Part model, mm, in its own coordinate system. Face numbers are marked on the shaded views. A direction names the side the tool comes from. Give positions to 0.01 mm unless a question says otherwise; leave off trailing zeros. Order: outer loops, then holes, each group sorted by start corner. A loop starts at its lowest first (then second) coordinate and runs counter-clockwise, first axis right, second up. Notation, with made-up numbers: M -30.5,88.25 L -20.5,88.25 A28 cw -20.5,125.25 Z; hole C 55.25,34 d2. An arc over 180 degrees is marked long. One line per question, with ' | ' between items.
```python
from build123d import *

# Parameters (mm, degrees)
SKETCH_1_R             = 5.5
EXTRUDE_1_DEPTH        = 68
CHAMFER_1_SIZE         = 0.5
SKETCH_2_R             = 3.3
EXTRUDE_2_DEPTH        = 8
HOLE_WIZARD_M5_1_D     = 4.2
HOLE_WIZARD_M5_1_DEPTH = 12.4
HOLE_WIZARD_M5_1_TIP   = 1.2618073
CHAMFER_3_SIZE         = 0.5
SKETCH_6_W             = 10
SKETCH_6_H             = 3
CUT_EXTRUDE_1_DEPTH    = 13


# Read off the part's stored shape, not the designer's step: M6 机械螺纹 螺柱1
with BuildPart() as part:
    # 草图1 → 拉伸1 (new body)
    with BuildSketch(Plane.XY):
        Circle(SKETCH_1_R)
    extrude(amount=EXTRUDE_1_DEPTH)

    # 倒角1
    chamfer_1_edges = [part.edges().sort_by_distance(p)[0] for p in [
        (-5.5, 0, 0),
        (-5.5, 0, 68),
    ]]
    chamfer(chamfer_1_edges, length=CHAMFER_1_SIZE)

    # 草图2 → 拉伸2 (add)
    with BuildSketch(Plane.XY.offset(68)):
        Circle(SKETCH_2_R)
    extrude(amount=EXTRUDE_2_DEPTH)

    # M5 螺纹孔1
    with Locations(Plane(origin=(0, 0, 0), x_dir=(-1, 0, 0), z_dir=(0, 0, -1))):
        with Locations((0, 0)):
            Hole(HOLE_WIZARD_M5_1_D / 2, depth=HOLE_WIZARD_M5_1_DEPTH)
            with Locations((0, 0, -(HOLE_WIZARD_M5_1_DEPTH + HOLE_WIZARD_M5_1_TIP / 2))):  # 118° drill point
                Cone(0, HOLE_WIZARD_M5_1_D / 2, HOLE_WIZARD_M5_1_TIP, mode=Mode.SUBTRACT)

    # 倒角3
    chamfer_3_edges = [part.edges().sort_by_distance(p)[0] for p in [
        (-2.1, 0, 0),
    ]]
    chamfer(chamfer_3_edges, length=CHAMFER_3_SIZE)

    # 草图6 → 切除-拉伸1 (cut)
    with BuildSketch(Plane(origin=(0, 0, 0), x_dir=(-1, 0, 0), z_dir=(0, 0, -1))):
        with Locations((0, 6.5)):
            Rectangle(SKETCH_6_W, SKETCH_6_H)
        with Locations((0, -6.5)):
            Rectangle(SKETCH_6_W, SKETCH_6_H)
    extrude(amount=-CUT_EXTRUDE_1_DEPTH, mode=Mode.SUBTRACT)

    # M6 机械螺纹 螺柱1 outline → M6 机械螺纹 螺柱1 (revolve, cut)
    with BuildSketch(Plane.XZ):
        Polygon((3.3, 76), (2.4585, 76), (3, 75.4585), (3, 68), (3.3, 68), align=None)
    revolve(axis=Axis((0, 0, 0), (0, 0, 1)), mode=Mode.SUBTRACT)


solid = part.part
```
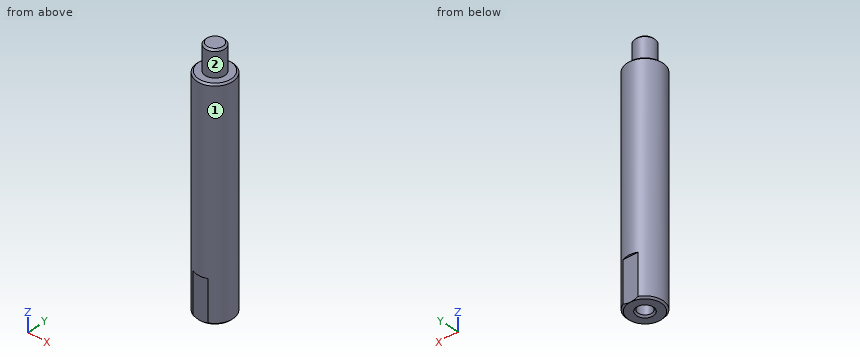
1. Probe L1, parallel to X at y = 0, z = 9.75; L2, parallel to Y at x = 5, z = 28.5; L3, parallel to Z at x = 2.75, y = -2. List the from-to ranges inside material, lowest first. Write a range as from..to.
Worked out:
L1: x = -5.5..-2.1, 2.1..5.5 | L2: y = -2.29..2.29 | L3: z = 0..68
2. Tool access for the marked faces 1 and 2: list every direction of +Z, -Z, +X, -X, +Y, -Y with a clear straight run to the whole face (end or side of a thin tool).
Worked out:
face 1: +Z, -Z | face 2: +Z
3. Drop flat-ended pins along their axis: pin 1 (4 mm diameter, centred on x = -3.5, y = 4.5, fed in from -Z); pin 2 (1 mm diameter, centred on x = 4.5, z = 45, fed in from +Y); pin 3 (3.5 mm diameter, centred on x = 0.5, z = 8.5, fed in from -Y); pin 4 (1.5 mm diameter, centred on y = 4, z = 33.5, fed in from -X). Give the stop position or say it passes through.
Worked out:
pin 1: stops at z = 0 | pin 2: stops at y = 3.77 | pin 3: stops at y = -5 | pin 4: stops at x = -4.44
4. Slice it at B-B on z = 24. Give the cut face in (x, y).
Worked out:
outline: C 0,0 d11
5. Slice it at A-A on z = 11.5. Give the cut face in (x, y), then the cut area to 3 significant figures.
Worked out:
outline: M -2.29,-5 L 2.29,-5 A5.5 ccw 2.29,5 L -2.29,5 A5.5 ccw Z; hole C 0,0 d4.2 | area: 78.1 mm2
